Design review of the part built by this model. Coordinates are the model's own, in mm. A direction names the side the tool comes from. Give positions to 0.01 mm unless a question says otherwise; leave off trailing zeros. Order: outer loops, then holes, each group sorted by start corner. A loop starts at its lowest first (then second) coordinate and runs counter-clockwise, first axis right, second up. Notation, with made-up numbers: (49, 72.5) -> (104, 72.5) arc R17 cw to (104, 82.5) -> close; hole circle Ø3 at (71, 69.5). An arc over 180 degrees is marked (long way). Use a Markdown table: item, result. Add a question column.
```python
from build123d import *

# Parameters (mm, degrees)
SKETCH_1_R          = 5.5
EXTRUDE_1_DEPTH     = 26
SKETCH_2_W          = 8
SKETCH_2_H          = 18
CUT_EXTRUDE_1_DEPTH = 25
SKETCH_3_R          = 1.5
CUT_EXTRUDE_2_DEPTH = 25
CUT_EXTRUDE_3_DEPTH = 11
SKETCH_6_W          = 25.84971197
SKETCH_6_H          = 26.022962568
SKETCH_6_W_2        = 3
SKETCH_6_H_2        = 6
CUT_EXTRUDE_4_DEPTH = 15


with BuildPart() as part:
    # 草图1 → 凸台-拉伸1 (new body)
    with BuildSketch(Plane(origin=(0, 0, 0), x_dir=(1, 0, 0), z_dir=(0, 1, 0))):
        Circle(SKETCH_1_R)
    extrude(amount=EXTRUDE_1_DEPTH)

    # 草图2 → 切除-拉伸1 (cut, symmetric)
    with BuildSketch(Plane.XY):
        with Locations((0, 26)):
            Rectangle(SKETCH_2_W, SKETCH_2_H)
    extrude(amount=CUT_EXTRUDE_1_DEPTH, both=True, mode=Mode.SUBTRACT)

    # 草图3 → 切除-拉伸2 (cut, symmetric)
    with BuildSketch(Plane(origin=(-4, 0, 0), x_dir=(0, 0, -1), z_dir=(1, 0, 0))):
        with Locations((0, 23)):
            Circle(SKETCH_3_R)
    extrude(amount=CUT_EXTRUDE_2_DEPTH, both=True, mode=Mode.SUBTRACT)

    # 草图5 → 切除-拉伸3 (cut, symmetric)
    with BuildSketch(Plane(origin=(0, 0, 0), x_dir=(0, 0, -1), z_dir=(1, 0, 0))):
        with BuildLine():
            Line((-4.153311931, 21.5), (-12.215121886, 24.91830584))
            Line((-12.215121886, 24.91830584), (0.629850505, 32.78071868))
            Line((0.629850505, 32.78071868), (12.991410006, 24.598657791))
            Line((12.991410006, 24.598657791), (4.153311931, 21.5))
            ThreePointArc((4.153311931, 21.5), (0, 25.653311931), (-4.153311931, 21.5))
        make_face()
    extrude(amount=CUT_EXTRUDE_3_DEPTH, both=True, mode=Mode.SUBTRACT)

    # 草图6 → 切除-拉伸4 (cut)
    with BuildSketch(Plane(origin=(0, 0, 0), x_dir=(-1, 0, 0), z_dir=(0, -1, 0))):
        Rectangle(SKETCH_6_W, SKETCH_6_H)
        Rectangle(SKETCH_6_W_2, SKETCH_6_H_2, mode=Mode.SUBTRACT)
    extrude(amount=-CUT_EXTRUDE_4_DEPTH, mode=Mode.SUBTRACT)


solid = part.part
```
1) Add section A-A (z = 0). Give the boundary of the cut face in (x, y), then the cut area to 3 significant figures.
2) Add section C-C (x = 0). Give the boundary of the cut face in (y, z).
3) For L1, parallel to Y at x = -4.9, z = 0; L2, parallel to X at y = 3.5, z = 1.25; L3, parallel to Z at x = -4.45, y = 23, list the stretches that pass through material, from the lowest coordinate up. Write a range as [from, to].
4) Machinability: for faces 1 (the flat face through (-1.5, 7, 0)), 2 (the flat face through (-4, 20, 0)), 3 (the flat face through (0, 7, -3)), which of the approach directions +Z, -Z, +X, -X, +Y, -Y give a long, thin tool a straight path to every point of the face, cutting with its end or side? Answer none if there is none.
5) Add section D-D (z = 1.75). Give the boundary of the cut face in (x, y).
6) Add section B-B (y = 22.5). Give the boundary of the cut face in (x, z).
7) The part is to be moulded in two halves that separate along Y. For faces 4 (the cylindrical face through (-4.74, 23.45, -1.43)), 5 (the flat face through (4, 20, 0)), 6 (the flat face through (0, 17, 0)), say which applies: +Y half, -Y half, draft (parallel to the pull), parting line (faces both ways), or undercut.
8) Insertion check: pin 1 (2 mm diameter, centred on x = -2, z = 2.5, fed in from +Y); pin 2 (3 mm diameter, centred on x = -1.5, y = 11.5, fed in from +Z); pin 3 (5 mm diameter, centred on y = 9.5, z = -3, fed in from -X). Each pin has a flat end and moves straight along its axis. Give the tip position at first contact, or say it passes through.
Worked answers:
| question | item | result |
|---|---|---|
| 1 | outline | (-5.5, 15) -> (-1.5, 15) -> (-1.5, 0) -> (1.5, 0) -> (1.5, 15) -> (5.5, 15) -> (5.5, 21.5) -> (4, 21.5) -> (4, 17) -> (-4, 17) -> (-4, 21.5) -> (-5.5, 21.5) -> close; (-5.5, 24.5) -> (-4, 24.5) -> (-4, 25.65) -> (-5.5, 25.65) -> close; (4, 24.5) -> (5.5, 24.5) -> (5.5, 25.65) -> (4, 25.65) -> close |
| 1 | area | 84.0 mm^2 |
| 2 | outline | (0, -3) -> (15, -3) -> (15, -5.5) -> (17, -5.5) -> (17, 5.5) -> (15, 5.5) -> (15, 3) -> (0, 3) -> close |
| 3 | L1 | [15, 21.5], [24.5, 25.65] |
| 3 | L2 | [-1.5, 1.5] |
| 3 | L3 | [-3.23, -1.5], [1.5, 3.23] |
| 4 | face 1 | +Z, -Z, -X, -Y |
| 4 | face 2 | +Z, -Z, +Y |
| 4 | face 3 | -Z, +X, -X, -Y |
| 5 | outline | (-5.21, 15) -> (-1.5, 15) -> (-1.5, 0) -> (1.5, 0) -> (1.5, 15) -> (5.21, 15) -> (5.21, 25.27) -> (4, 25.27) -> (4, 17) -> (-4, 17) -> (-4, 25.27) -> (-5.21, 25.27) -> close |
| 6 | outline | (-5.32, -1.41) arc R5.5 ccw to (-4, -3.77) -> (-4, -1.41) -> close; (-5.32, 1.41) -> (-4, 1.41) -> (-4, 3.77) arc R5.5 ccw to start; (4, -3.77) arc R5.5 ccw to (5.32, -1.41) -> (4, -1.41) -> close; (4, 1.41) -> (5.32, 1.41) arc R5.5 ccw to (4, 3.77) -> close |
| 7 | face 4 | undercut |
| 7 | face 5 | draft |
| 7 | face 6 | +Y half |
| 8 | pin 1 | y = 17 |
| 8 | pin 2 | z = 3 |
| 8 | pin 3 | x = -1.5 |
